Autodesk Inventor part; units mm, degrees
ref_plane "YZ Plane" through (0, 0, 0) normal (1, 0, 0) x (0, 1, 0)
ref_plane "XZ Plane" through (0, 0, 0) normal (0, 1, 0) x (-1, 0, 0)
ref_plane "XY Plane" through (0, 0, 0) normal (0, 0, 1) x (1, 0, 0)
sketch "Sketch1" plane through (0, 0, 0) normal (0, 1, 0) x (-1, 0, 0)
  line L0 (0, 0) -> (36, 0)
  line L1 (36, 0) -> (36, -80)
  line L2 (36, -80) -> (0, -80)
  line L3 (0, -80) -> (0, 0)
  circle A0 centre (33.85, -77.85) radius 1.35
  circle A1 centre (2.15, -77.85) radius 1.35
  circle A2 centre (33.85, -2.15) radius 1.35
  circle A3 centre (2.15, -2.15) radius 1.35
  dimension "d0" = 36
  dimension "d1" = 80
  dimension "d2" = 2.7
  dimension "d3" = 2.15
  dimension "d4" = 2.15
  dimension "d5" = 2.7
  dimension "d6" = 2.15
  dimension "d7" = 2.7
  dimension "d8" = 2.15
  dimension "d9" = 2.7
extrude "Extrusion1" add sketch "Sketch1" along normal blind 1.6
sketch "Sketch2" plane through (0, 1.6, 0) normal (0, 1, 0) x (1, 0, 0)
  line L0 (-29.35, 4.5) -> (-5, 4.5)
  line L1 (-5, 4.5) -> (-5, 75.7)
  line L2 (-5, 75.7) -> (-29.35, 75.7)
  line L3 (-29.35, 75.7) -> (-29.35, 4.5)
  line L4 (-36, 0) -> (0, 0)
  line L5 (0, 0) -> (0, 80)
  dimension "d12" = 24.35
  dimension "d13" = 71.2
  dimension "d14" = 4.5
  dimension "d15" = 5
extrude "Extrusion2" add sketch "Sketch2" along normal blind 6.25
sketch "Sketch3" plane through (0, 1.6, 0) normal (0, 1, 0) x (1, 0, 0)
  line L0 (-34, 7.1651) -> (-33, 7.1651)
  line L1 (-33, 7.1651) -> (-33, 46.1651)
  line L2 (-33, 46.1651) -> (-34, 46.1651)
  line L3 (-34, 46.1651) -> (-34, 7.1651)
  line L4 (-36, 80) -> (-36, 0)
  point P0 (0, 0)
  dimension "d18" = 1
  dimension "d19" = 39
  dimension "d20" = 2
extrude "Extrusion3" add sketch "Sketch3" along normal blind 3.6
sketch "Sketch4" plane through (-5, 1.6, -75.7) normal (0, 0, -1) x (-1, 0, 0)
  line L0 (-5, 0) -> (31, 0)
  line L1 (2.5, 0) -> (21.85, 0)
  line L2 (21.85, 0) -> (21.85, 2.3329)
  line L3 (21.85, 2.3329) -> (2.5, 2.3329)
  line L4 (2.5, 2.3329) -> (2.5, 0)
  line L5 (0, 0) -> (0, 6.25)
  line L6 (24.35, 0) -> (24.35, 6.25)
  point P0 (-5, -1.6)
  dimension "d23" = 2.5
  dimension "d24" = 2.5
extrude "Extrusion4" add sketch "Sketch4" along normal blind 3.6
sketch "Sketch5" plane through (-26.85, 3.9329, -75.7) normal (0, 1, 0) x (1, 0, 0)
  line L0 (19.35, 0) -> (15.75, 3.6)
  line L1 (19.35, 0) -> (24.4412, 0) construction
  line L2 (0, 0) -> (3.6, 3.6)
  line L3 (0, 0) -> (5.0912, 0) construction
  line L4 (3.6, 3.6) -> (15.75, 3.6)
  line L5 (19.35, 3.6) -> (19.35, 0)
  line L6 (19.35, 0) -> (19.35, 3.6)
  line L7 (19.35, 3.6) -> (15.75, 3.6)
  line L8 (3.6, 3.6) -> (0, 3.6)
  line L9 (0, 0) -> (0, 3.6)
  line L10 (21.85, 0) -> (-2.5, 0)
  point P0 (26.85, -75.7)
  dimension "d27" = 135
  dimension "d28" = 45
extrude "Extrusion5" cut sketch "Sketch5" against normal blind 2.333 contours L0 L7 L5 | L9 L8 L2
sketch "Sketch6" plane through (0, 0, 0) normal (0, -1, 0) x (1, 0, 0)
  line L0 (-34.5, -6) -> (-15.15, -6)
  line L1 (-15.15, -6) -> (-15.15, -48)
  line L2 (-15.15, -48) -> (-34.5, -48)
  line L3 (-34.5, -48) -> (-34.5, -6)
  line L4 (-36, 0) -> (-36, -80)
  line L5 (0, 0) -> (-36, 0)
  dimension "d31" = 19.35
  dimension "d32" = 42
  dimension "d33" = 1.5
  dimension "d34" = 6
extrude "Extrusion6" add sketch "Sketch6" along normal blind 4.15
sketch "Sketch7" plane through (0, -4.15, 0) normal (0, -1, 0) x (1, 0, 0)
  line L0 (-15.15, -6) -> (-34.5, -6)
  line L1 (-29.5, -6) -> (-19.1, -6)
  line L2 (-19.1, -6) -> (-19.1, -8.4)
  line L3 (-19.1, -8.4) -> (-29.5, -8.4)
  line L4 (-29.5, -8.4) -> (-29.5, -6)
  line L5 (-34.5, -6) -> (-34.5, -48)
  point P0 (0, 0)
  dimension "d37" = 10.4
  dimension "d38" = 2.4
  dimension "d39" = 5
extrude "Extrusion7" add sketch "Sketch7" along normal blind 5.5
sketch "Sketch8" plane through (-34.5, 0, -6) normal (0, 0, 1) x (1, 0, 0)
  line L0 (15.4, -9.65) -> (5, -9.65)
  line L1 (15.4, -4.15) -> (15.4, -9.65)
  line L2 (5, -9.65) -> (15.4, -9.65)
  line L3 (15.4, -9.65) -> (15.4, -7)
  line L4 (15.4, -7) -> (5, -7)
  line L5 (5, -7) -> (5, -9.65)
  point P0 (34.5, 0)
  dimension "d42" = 2.65
extrude "Extrusion8" add sketch "Sketch8" along normal blind 10.75
properties part number "LCD_Screen"
Verification items for the finished model (mm, model axes). A direction names the side the tool comes from. Round coordinates to 2 decimals unless told otherwise and drop trailing zeros. Write each loop counter-clockwise with the first axis right and the second up, starting at its lowest first coordinate (ties: lowest second). Pieces come first, ordered by that corner, then holes. Notation, with made-up numbers: (80.25, -16) - (121.25, -16) arc R22 cw to (121.25, 23) - close; hole circle Ø5 at (-13.75, 68). An arc over 180 degrees is marked (long way). Answer as a JSON object with one key per item and string values. Group by question number.
Q1. Tool access check on faces 1 (the flat face through (-24, -7, -1)), 2 (the flat face through (-25, 1.6, -78)), 3 (the flat face through (-17, 3, -79.3)). Record the directions out of +Z, -Z, +X, -X, +Y, -Y that give a thin tool (end or side, any length) a straight path to the whole face; none if there is none.
Q2. Section check C-C, the plane z = -77.85. Give the number of separate pieces and of enclosed holes in the cut face, plus the area to 3 significant figures.
Q3. Go/stop test with flat-tipped pins: pin 1 Ø3 at (x, y) = (-30.5, -4) entering from -Z; pin 2 Ø4 at (x, z) = (-16.5, -39.5) entering from -Y; pin 3 Ø1.5 at (y, z) = (-5.5, -18.5) entering from +X; pin 4 Ø1.5 at (x, y) = (-24, 5) entering from -Z. Record where each tip stops, or that it passes through.
Q4. Section check B-B, the plane x = -2.15. Enter the section's corners in (y, z), plus the area to 3 significant figures.
Q5. Section check A-A, the plane z = -2.15. Enter the section's corners in (x, y).
Q6. Thickness scan on line 1 (Z direction, x = -2.15, y = 0.7); line 2 (X direction, y = 5, z = -19.5); line 3 (X direction, y = 1.1, z = -77.85). Record the ranges inside material, lowest first.
Q7. Mould release check, pull along Z, two halves, no side actions. Record for faces 4 (the flat face through (-24, -8, 4.75)), 5 (the cylindrical face through (-1.974, 0.789, -79.189)), 6 (the flat face through (-9, 1.6, -78)): released by +Z, released by -Z, zero draft, split by the parting line, or undercut.
Q8. Section check D-D, the plane x = -16.5. Enter the section's corners in (y, z).
Found:
{
 "1": {"face 1": "+Z, +X, -X", "face 2": "-Z, -X, +Y", "face 3": "-Z, +X, -X, +Y"},
 "2": {"separate pieces": "3", "enclosed holes": "0", "area": "84.1 mm^2"},
 "3": {"pin 1": "stops at z = -48", "pin 2": "stops at y = -4.15", "pin 3": "passes through", "pin 4": "stops at z = -75.7"},
 "4": {"outline": "(0, -80) - (1.6, -80) - (1.6, -79.2) - (0, -79.2) - close; (0, -76.5) - (1.6, -76.5) - (1.6, -3.5) - (0, -3.5) - close; (0, -0.8) - (1.6, -0.8) - (1.6, 0) - (0, 0) - close", "area": "119 mm^2"},
 "5": {"outline": "(-36, 0) - (-35.2, 0) - (-35.2, 1.6) - (-36, 1.6) - close; (-32.5, 0) - (-3.5, 0) - (-3.5, 1.6) - (-32.5, 1.6) - close; (-29.5, -9.65) - (-19.1, -9.65) - (-19.1, -7) - (-29.5, -7) - close; (-0.8, 0) - (0, 0) - (0, 1.6) - (-0.8, 1.6) - close"},
 "6": {"line 1": "z = -80 to -79.2, -76.5 to -3.5, -0.8 to 0", "line 2": "x = -34 to -33, -29.35 to -5", "line 3": "x = -36 to -35.2, -32.5 to -3.5, -0.8 to 0"},
 "7": {"face 4": "released by +Z", "face 5": "undercut", "face 6": "zero draft"},
 "8": {"outline": "(-4.15, -48) - (0, -48) - (0, -80) - (1.6, -80) - (1.6, -79.3) - (3.93, -79.3) - (3.93, -75.7) - (7.85, -75.7) - (7.85, -4.5) - (1.6, -4.5) - (1.6, 0) - (0, 0) - (0, -6) - (-4.15, -6) - close"}
}
